Autodesk Inventor part; units mm, degrees
ref_plane "YZ Plane" through (0, 0, 0) normal (1, 0, 0) x (0, 1, 0)
ref_plane "XZ Plane" through (0, 0, 0) normal (0, 1, 0) x (-1, 0, 0)
ref_plane "XY Plane" through (0, 0, 0) normal (0, 0, 1) x (1, 0, 0)
sketch "Sketch15" plane through (0, 0, 0) normal (0, 1, 0) x (-1, 0, 0)
  line L0 (0, 0) -> (203.2, 0)
  line L1 (203.2, 0) -> (203.2, -203.2)
  line L2 (203.2, -203.2) -> (0, -203.2)
  line L3 (0, -203.2) -> (0, 0)
  dimension "d149" = 203.2
  dimension "d150" = 203.2
extrude "Extrusion15" add sketch "Sketch15" along normal blind 76.2
sketch "Sketch16" plane through (0, 76.2, 0) normal (0, 1, 0) x (1, 0, 0)
  line L0 (-166.6, 166.6) -> (-36.6, 166.6)
  line L1 (-36.6, 166.6) -> (-36.6, 36.6)
  line L2 (-36.6, 36.6) -> (-166.6, 36.6)
  line L3 (-166.6, 36.6) -> (-166.6, 166.6)
  line L4 (0, 0) -> (0, 203.2)
  dimension "d153" = 130
  dimension "d154" = 130
  dimension "d155" = 36.6
  dimension "d156" = 36.6
extrude "Extrusion16" cut sketch "Sketch16" against normal through all
sketch "Sketch17" plane through (-203.2, 0, 0) normal (0, 0, 1) x (1, 0, 0)
  line L0 (203.2, 0) -> (0, 0)
  line L1 (0, 0) -> (0, 38.1)
  line L2 (0, 38.1) -> (101.6, 38.1)
  circle A0 centre (116.84, 38.1) radius 3.175
  circle A1 centre (101.6, 53.34) radius 3.175
  circle A2 centre (86.36, 38.1) radius 3.175
  circle A3 centre (101.6, 22.86) radius 3.175
  dimension "d159" = 101.6
  dimension "d160" = 38.1
  dimension "d161" = 6.35
  dimension "d162" = 15.24
  dimension "d163" = 0
  dimension "d166" = 360
extrude "Extrusion17" cut sketch "Sketch17" against normal blind 101.6
sketch "Sketch19" plane through (0, 76.2, 0) normal (0, 1, 0) x (1, 0, 0)
  line L0 (-36.6, 36.6) -> (-36.6, 166.6)
  line L1 (-36.6, 121.6) -> (0.103, 121.6)
  line L2 (0.103, 121.6) -> (0.103, 81.6)
  line L3 (0.103, 81.6) -> (-36.6, 81.6)
  line L4 (-36.6, 81.6) -> (-36.6, 121.6)
  line L5 (-166.6, 166.6) -> (-36.6, 166.6)
  point P0 (0, 0)
  dimension "d170" = 40
  dimension "d171" = 45
  dimension "d172" = 36.703
sketch "Sketch22" plane through (0, 76.2, 0) normal (0, 1, 0) x (1, 0, 0)
  line L0 (-166.6, 36.6) -> (-166.6, 62.6)
  line L1 (-166.6, 36.6) -> (-140.6, 36.6)
  line L2 (-140.6, 36.6) -> (-140.6, 50.487)
  line L3 (-166.6, 62.6) -> (-152.713, 62.6)
  arc A0 (-152.713, 62.6) -> (-140.6, 50.487) centre (-100.3536, 102.8464) ccw
  circle A1 centre (-153.25, 49.835) radius 4.4958
  line L4 (-166.6, 166.6) -> (-166.6, 140.6)
  line L5 (-166.6, 166.6) -> (-140.6, 166.6)
  line L6 (-166.6, 140.6) -> (-152.713, 140.6)
  line L7 (-140.6, 166.6) -> (-140.6, 152.713)
  arc A2 (-140.6, 152.713) -> (-152.713, 140.6) centre (-100.3536, 100.3536) ccw
  circle A3 centre (-153.25, 153.365) radius 4.4958
  line L8 (-101.6, 36.6) -> (-101.6, 166.6)
  line L9 (-166.6, 166.6) -> (-140.6, 166.6)
  line L10 (-166.6, 140.6) -> (-166.6, 166.6)
  line L11 (-166.6, 36.6) -> (-140.6, 36.6)
  line L12 (-166.6, 166.6) -> (-166.6, 140.6)
  line L13 (-36.6, 36.6) -> (-36.6, 62.6)
  line L14 (-36.6, 36.6) -> (-62.6, 36.6)
  line L15 (-62.6, 36.6) -> (-62.6, 50.487)
  line L16 (-36.6, 62.6) -> (-50.487, 62.6)
  arc A4 (-62.6, 50.487) -> (-50.487, 62.6) centre (-102.8464, 102.8464) ccw
  circle A5 centre (-49.95, 49.835) radius 4.4958
  line L17 (-36.6, 166.6) -> (-36.6, 140.6)
  line L18 (-36.6, 166.6) -> (-62.6, 166.6)
  line L19 (-36.6, 140.6) -> (-50.487, 140.6)
  line L20 (-62.6, 166.6) -> (-62.6, 152.713)
  arc A6 (-50.487, 140.6) -> (-62.6, 152.713) centre (-102.8464, 100.3536) ccw
  circle A7 centre (-49.95, 153.365) radius 4.4958
  point P0 (0, 0)
  dimension "d191" = 26
  dimension "d206" = 13.887
  dimension "d207" = 13.887
  dimension "d208" = 66.04
  dimension "d210" = 13.35
  dimension "d214" = 8.9916
  dimension "d217" = 12.765
  dimension "d218" = 26
  dimension "d219" = 26
  dimension "d220" = 13.887
  dimension "d221" = 13.887
  dimension "d222" = 66.04
  dimension "d223" = 8.9916
  dimension "d224" = 12.765
  dimension "d225" = 13.35
  dimension "d232" = 90
  dimension "d233" = 26
  dimension "d234" = 65
  dimension "d235" = 130
  dimension "d236" = 0
sketch "Sketch23" plane through (0, 0, -203.2) normal (0, 0, -1) x (-1, 0, 0)
  line L0 (0, 0) -> (0, 38.1)
  circle A0 centre (127, 38.1) radius 3.175
  line L1 (0, 38.1) -> (101.6, 38.1)
  circle A1 centre (101.6, 63.5) radius 3.175
  circle A2 centre (76.2, 38.1) radius 3.175
  circle A3 centre (101.6, 12.7) radius 3.175
  dimension "d180" = 101.6
  dimension "d181" = 38.1
  dimension "d182" = 25.4
  dimension "d183" = 0
  dimension "d184" = 6.35
  dimension "d187" = 360
extrude "Extrusion20" cut sketch "Sketch23" against normal blind 101.6
extrude "Extrusion28" add sketch "Sketch22" against normal blind 76.2
sketch "Sketch26" plane through (0, 76.2, 0) normal (0, 1, 0) x (1, 0, 0)
  line L0 (-62.6, 166.6) -> (-140.6, 166.6)
  line L1 (-140.6, 166.6) -> (-140.6, 174.22)
  line L2 (-140.6, 174.22) -> (-62.6, 174.22)
  line L3 (-62.6, 174.22) -> (-62.6, 166.6)
  line L4 (-140.6, 152.713) -> (-140.6, 166.6)
  line L5 (-140.6, 36.6) -> (-140.6, 50.487)
  line L6 (-140.6, 36.6) -> (-62.6, 36.6)
  line L7 (-62.6, 36.6) -> (-62.6, 28.98)
  line L8 (-62.6, 28.98) -> (-140.6, 28.98)
  line L9 (-140.6, 28.98) -> (-140.6, 36.6)
  line L10 (-62.6, 50.487) -> (-62.6, 36.6)
  point P0 (0, 0)
  dimension "d242" = 0
  dimension "d243" = 7.62
  dimension "d244" = 0
  dimension "d245" = 7.62
extrude "Extrusion29" cut sketch "Sketch26" against normal through all
sketch "Sketch28" plane through (0, 76.2, 0) normal (0, 1, 0) x (1, 0, 0)
  line L0 (-166.6, 140.6) -> (-166.6, 62.6)
  line L1 (-166.6, 140.6) -> (-174.22, 140.6)
  line L2 (-174.22, 140.6) -> (-174.22, 62.6)
  line L3 (-174.22, 62.6) -> (-166.6, 62.6)
  line L4 (-166.6, 62.6) -> (-166.6, 140.6)
  line L5 (-152.713, 62.6) -> (-166.6, 62.6)
  line L6 (-36.6, 62.6) -> (-36.6, 140.6)
  line L7 (-36.6, 62.6) -> (-28.98, 62.6)
  line L8 (-28.98, 62.6) -> (-28.98, 140.6)
  line L9 (-28.98, 140.6) -> (-36.6, 140.6)
  line L10 (-36.6, 140.6) -> (-36.6, 62.6)
  line L11 (-50.487, 140.6) -> (-36.6, 140.6)
  point P0 (0, 0)
  point P1 (-170.41, 62.6)
  dimension "d253" = 0
  dimension "d254" = 7.62
  dimension "d255" = 0
  dimension "d256" = 7.62
extrude "Extrusion30" cut sketch "Sketch28" against normal through all
fillet "Fillet9" radius 6.35 8 edges at (-140.6, 38.1, -174.22) (-62.6, 38.1, -174.22) (-28.98, 38.1, -140.6) (-28.98, 38.1, -62.6) (-62.6, 38.1, -28.98) (-140.6, 38.1, -28.98) (-174.22, 38.1, -62.6) (-174.22, 38.1, -140.6)
extrude "Extrusion31" cut sketch "Sketch19" against normal through all
properties part number "FrontPlateV2"
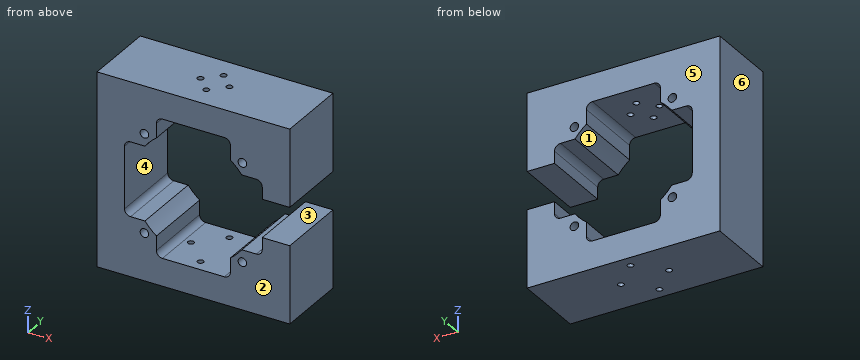
Geometry check sheet. Reference: the model listing, model coordinates, mm. Face numbers are marked on the shaded views. A direction names the side the tool comes from. Round coordinates to 2 decimals unless told otherwise and drop trailing zeros. Loops run counter-clockwise (first coordinate to the right, second up) from the corner with the lowest first, then second, coordinate; pieces in that order, holes last. Notation, with made-up numbers: (3, 34) - (27, 34) arc R23 cw to (27, 59) - close; hole circle Ø1 at (38, 49.25). An arc over 180 degrees is marked (long way). Write item = value, one per line. Start each with the question number.
1. Section check C-C on x = -127. Enter the section's corners in (y, z) (3 decimals).
2. Thickness scan on line 1 (Y direction, x = -101, z = -23); line 2 (Z direction, x = -153.25, y = 20.5); line 3 (Z direction, x = -159, y = 34.5). Record the ranges inside material, lowest first.
3. Depth check by flat-ended pin: pin 1 (7 mm diameter, centred on x = -49.95, z = -153.365, fed in from -Y); pin 2 (5.5 mm diameter, centred on x = -101.6, y = 53.34, fed in from +Z); pin 3 (1 mm diameter, centred on y = 21.5, z = -88.5, fed in from +X). Enter the tip coordinate at first touch or a pass-through.
4. Section check D-D on y = 38.1. Give the number of separate pieces and of enclosed holes in the cut face, then the cut area to 3 significant figures.
5. Set-up check for the marked faces 1, 2 and 3: record each of +Z, -Z, +X, -X, +Y, -Y from which the full face is reachable in a straight line by a thin tool's end or side.
6. Section check A-A on x = -164. Enter the section's corners in (y, z), then the cut area to 3 significant figures.
7. Mould release check, pull along X, two halves, no side actions. Record for the marked faces 4, 5 and 6: released by +X, released by -X, zero draft, split by the parting line, or undercut.
8. Section check B-B on z = -130. Enter the section's corners in (x, y).
Working result:
q1.outline = (0, -203.2) - (34.925, -203.2) - (34.925, -174.22) - (0, -174.22) - close; (0, -28.98) - (76.2, -28.98) - (76.2, 0) - (0, 0) - close; (41.275, -203.2) - (76.2, -203.2) - (76.2, -174.22) - (41.275, -174.22) - close
q2.line_1 = 0 to 19.74, 25.98 to 50.22, 56.46 to 76.2
q2.line_2 = -203.2 to -157.86, -148.87 to -140.6, -62.6 to -54.33, -45.34 to 0
q2.line_3 = -203.2 to -140.6, -62.6 to 0
q3.pin_1 = through
q3.pin_2 = -174.22
q3.pin_3 = -174.22
q4.separate_pieces = 5
q4.enclosed_holes = 4
q4.area = 22,300 mm^2
q5.face_1 = +Y, -Y
q5.face_2 = +Z, -Z, +X, -X, -Y
q5.face_3 = +X, +Y, -Y
q6.outline = (0, -203.2) - (76.2, -203.2) - (76.2, -140.6) - (0, -140.6) - close; (0, -62.6) - (76.2, -62.6) - (76.2, 0) - (0, 0) - close
q6.area = 9,540 mm^2
q7.face_4 = undercut
q7.face_5 = zero draft
q7.face_6 = released by -X
q8.outline = (-203.2, 0) - (-174.22, 0) - (-174.22, 76.2) - (-203.2, 76.2) - close; (-28.98, 0) - (0, 0) - (0, 76.2) - (-28.98, 76.2) - close
